Check sheet for the drawn part. Datum: minimum x, y, z corner. Units: mm. Give positions to 0.01 mm unless a question says otherwise; leave off trailing zeros. Order: outer loops, then holes, each group sorted by start corner. A loop starts at its lowest first (then second) coordinate and runs counter-clockwise, first axis right, second up. Notation, with made-up numbers: (-13, 26.5) -> (22, 26.5) arc R17 ccw to (22, 37.5) -> close; hole circle Ø4 at (-24, 81.25). An arc over 180 degrees is marked (long way). Answer in a Markdown table with one row per item. Add a question column.
(1) Go/stop test with flat-tipped pins: pin 1 (2 mm diameter, centred on x = 87, z = 15, fed in from -Y); pin 2 (2 mm diameter, centred on x = 17.5, z = 22.5, fed in from +Y). Record where each tip stops, or that it passes through.
(2) Cross-section at B-B (y = 50). Record the cut outline in (x, z).
(3) Cross-section at C-C (z = 13.25). Record the cut outline in (x, y).
(4) Cross-section at D-D (x = 8). Record the cut outline in (y, z).
(5) Cross-section at A-A (z = 3.5). Record the cut outline in (x, y), then the cut area to 3 significant figures.
(6) Thickness scan on L1, parallel to Y at x = 50, z = 20.75; L2, parallel to Y at x = 59, z = 18; L3, parallel to X at y = 59.5, z = 20.25. Record the ranges inside material, lowest first. Write a range as [from, to].
(7) Release check for a two-part mould opening along X. For the marked faces 1, 2, 3 and 4 record: released by +X, released by -X, zero draft, split by the parting line, or undercut.
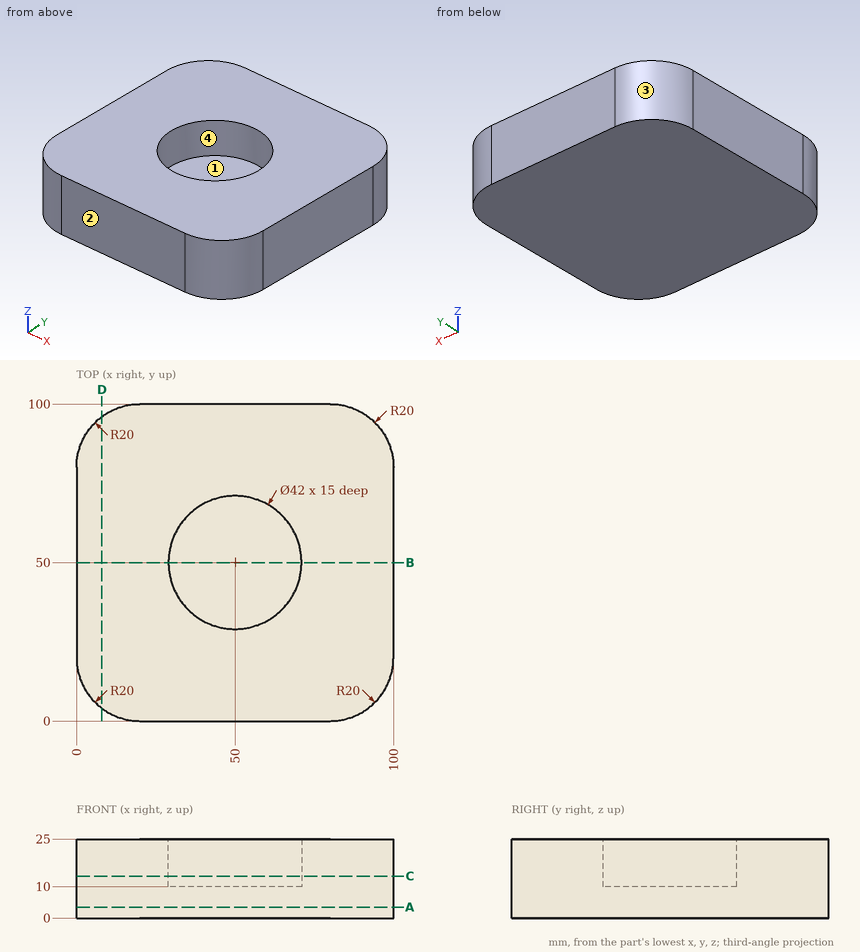
Answer below:
| question | item | result |
|---|---|---|
| 1 | pin 1 | stops at y = 0.92 |
| 1 | pin 2 | stops at y = 99.94 |
| 2 | outline | (0, 0) -> (100, 0) -> (100, 25) -> (71, 25) -> (71, 10) -> (29, 10) -> (29, 25) -> (0, 25) -> close |
| 3 | outline | (0, 20) arc R20 ccw to (20, 0) -> (80, 0) arc R20 ccw to (100, 20) -> (100, 80) arc R20 ccw to (80, 100) -> (20, 100) arc R20 ccw to (0, 80) -> close; hole circle Ø42 at (50, 50) |
| 4 | outline | (4, 0) -> (96, 0) -> (96, 25) -> (4, 25) -> close |
| 5 | outline | (0, 20) arc R20 ccw to (20, 0) -> (80, 0) arc R20 ccw to (100, 20) -> (100, 80) arc R20 ccw to (80, 100) -> (20, 100) arc R20 ccw to (0, 80) -> close |
| 5 | area | 9,660 mm² |
| 6 | L1 | y = [0, 29], [71, 100] |
| 6 | L2 | y = [0, 31.03], [68.97, 100] |
| 6 | L3 | x = [0, 31.27], [68.73, 100] |
| 7 | face 1 | undercut |
| 7 | face 2 | zero draft |
| 7 | face 3 | released by -X |
| 7 | face 4 | undercut |
